from build123d import *

# Parameters (mm, degrees)
SKETCH2_W               = 76.2
SKETCH2_H               = 50.8
BOSS_EXTRUDE2_DEPTH     = 3.175
CUT_EXTRUDE1_DEPTH      = 63.861792847
CUT_EXTRUDE1_DEPTH_BACK = 63.861792847
CUT_EXTRUDE3_START      = -3.175
CUT_EXTRUDE3_DEPTH      = 3.175
CUT_EXTRUDE2_DEPTH      = 77.530014537
CUT_EXTRUDE2_DEPTH_BACK = 15.24
SKETCH4_R               = 1.27


with BuildPart() as part:
    # Sketch2 → Boss-Extrude2 (new, symmetric)
    with BuildSketch(Plane(origin=(0, 0, 0), x_dir=(0, 0, -1), z_dir=(1, 0, 0))):
        Polygon((-57.15, -6.35), (-57.15, -25.4), (-38.1, -25.4), (-38.1, 25.4), align=None)
        Rectangle(SKETCH2_W, SKETCH2_H)
    extrude(amount=BOSS_EXTRUDE2_DEPTH, both=True)

    # Sketch3 → Cut-Extrude1 (cut, two sides: drawn at the far end of the back side and taken through both)
    with BuildSketch(Plane(origin=(3.175, 0, 0), x_dir=(0, 0, -1), z_dir=(1, 0, 0)).offset(-CUT_EXTRUDE1_DEPTH_BACK)):
        with BuildLine():
            Line((-12.499999952, -9.525), (-12.499999952, 15.875))
            ThreePointArc((-12.499999952, 15.875), (-14, 17.375000048), (-15.500000048, 15.875))
            Line((-15.500000048, 15.875), (-15.500000048, -9.525))
            ThreePointArc((-15.500000048, -9.525), (-14, -11.025000048), (-12.499999952, -9.525))
        make_face()
        with BuildLine():
            Line((15.500000048, -9.525), (15.500000048, 15.875))
            ThreePointArc((15.500000048, 15.875), (14, 17.375000048), (12.499999952, 15.875))
            Line((12.499999952, 15.875), (12.499999952, -9.525))
            ThreePointArc((12.499999952, -9.525), (14, -11.025000048), (15.500000048, -9.525))
        make_face()
    extrude(amount=CUT_EXTRUDE1_DEPTH + CUT_EXTRUDE1_DEPTH_BACK, mode=Mode.SUBTRACT)

    # Sketch3_3 → Cut-Extrude3 (cut)
    # profile 1 of 2: a face of its own
    with BuildSketch(Plane(origin=(3.175, 0, 0), x_dir=(0, 0, -1), z_dir=(1, 0, 0)).offset(CUT_EXTRUDE3_START)):
        with BuildLine():
            Line((-18.250000009, -9.525), (-18.250000009, 15.875))
            ThreePointArc((-18.250000009, 15.875), (-14, 20.125000009), (-9.749999991, 15.875))
            Line((-9.749999991, 15.875), (-9.749999991, -9.525))
            ThreePointArc((-9.749999991, -9.525), (-14, -13.775000009), (-18.250000009, -9.525))
        make_face()
        with BuildLine():
            Line((-15.500000048, -9.525), (-15.500000048, 15.875))
            ThreePointArc((-15.500000048, 15.875), (-14, 17.375000048), (-12.499999952, 15.875))
            Line((-12.499999952, 15.875), (-12.499999952, -9.525))
            ThreePointArc((-12.499999952, -9.525), (-14, -11.025000048), (-15.500000048, -9.525))
        make_face(mode=Mode.SUBTRACT)
    # profile 2 of 2: a face of its own
    with BuildSketch(Plane(origin=(3.175, 0, 0), x_dir=(0, 0, -1), z_dir=(1, 0, 0)).offset(CUT_EXTRUDE3_START)):
        with BuildLine():
            Line((9.749999991, -9.525), (9.749999991, 15.875))
            ThreePointArc((9.749999991, 15.875), (14, 20.125000009), (18.250000009, 15.875))
            Line((18.250000009, 15.875), (18.250000009, -9.525))
            ThreePointArc((18.250000009, -9.525), (14, -13.775000009), (9.749999991, -9.525))
        make_face()
        with BuildLine():
            Line((12.499999952, -9.525), (12.499999952, 15.875))
            ThreePointArc((12.499999952, 15.875), (14, 17.375000048), (15.500000048, 15.875))
            Line((15.500000048, 15.875), (15.500000048, -9.525))
            ThreePointArc((15.500000048, -9.525), (14, -11.025000048), (12.499999952, -9.525))
        make_face(mode=Mode.SUBTRACT)
    extrude(amount=CUT_EXTRUDE3_DEPTH, mode=Mode.SUBTRACT)

    # Sketch4 → Cut-Extrude2 (cut, two sides: drawn at the far end of the back side and taken through both)
    with BuildSketch(Plane.XZ.offset(25.4).offset(-CUT_EXTRUDE2_DEPTH_BACK)):
        with Locations(Location((0, 25.4, 0), (0, 0, 90))):
            Circle(SKETCH4_R)
        with Locations(Location((0, 0, 0), (0, 0, 90))):
            Circle(SKETCH4_R)
        with Locations(Location((0, -25.4, 0), (0, 0, 90))):
            Circle(SKETCH4_R)
        with Locations(Location((0, 34.925, 0), (0, 0, 90))):
            Circle(SKETCH4_R)
        with Locations(Location((0, 44.45, 0), (0, 0, 90))):
            Circle(SKETCH4_R)
    extrude(amount=CUT_EXTRUDE2_DEPTH + CUT_EXTRUDE2_DEPTH_BACK, mode=Mode.SUBTRACT)


solid = part.part
The model under review builds one solid part; all positions refer to its coordinate system, in mm. A direction names the side the tool comes from. Round coordinates to 2 decimals unless told otherwise and drop trailing zeros. Loops run counter-clockwise (first coordinate to the right, second up) from the corner with the lowest first, then second, coordinate; pieces in that order, holes last. Notation, with made-up numbers: M 77,15.25 L 86,15.25 A23 cw 86,27.25 Z; hole C 55,20.25 d7. An arc over 180 degrees is marked long. Answer as a JSON object with one key per item and string values.
Item 1: For line 1 along Z through (x, y) = (1, 13.5); line 2 along X through (y, z) = (-21, 0) (3 decimals); line 3 along Z through (x, y) = (2.25, 10), list the stretches that pass through material, from the lowest coordinate up.
Check sheet entries:
{"line 1": "-38.1 to -18.25, -9.75 to 9.75, 18.25 to 45.24", "line 2": "-3.175 to -1.27, 1.27 to 3.175", "line 3": "-38.1 to -18.25, -9.75 to 9.75, 18.25 to 47.34"}
Item 2: We need section C-C, the plane y = -20. State the section outline as (x, z) points (3 decimals).
Check sheet entries:
{"outline": "M -3.175,-38.1 L 3.175,-38.1 L 3.175,57.15 L -3.175,57.15 Z; hole C 0,-25.4 d2.54; hole C 0,0 d2.54; hole C 0,25.4 d2.54; hole C 0,34.925 d2.54; hole C 0,44.45 d2.54"}
Item 3: We need section B-B, the plane z = 14. State the section outline as (x, y) points (3 decimals).
Check sheet entries:
{"outline": "M -3.175,-25.4 L 3.175,-25.4 L 3.175,-13.775 L 0,-13.775 L 0,-11.025 L -3.175,-11.025 Z; M -3.175,17.375 L 0,17.375 L 0,20.125 L 3.175,20.125 L 3.175,25.4 L -3.175,25.4 Z"}
Item 4: We need section D-D, the plane y = -4. State the section outline as (x, z) points (3 decimals), and give its area (3 significant figures).
Check sheet entries:
{"outline": "M -3.175,-38.1 L 3.175,-38.1 L 3.175,-18.25 L 0,-18.25 L 0,-15.5 L -3.175,-15.5 Z; M -3.175,-12.5 L 0,-12.5 L 0,-9.75 L 3.175,-9.75 L 3.175,9.75 L 0,9.75 L 0,12.5 L -3.175,12.5 Z; M -3.175,15.5 L 0,15.5 L 0,18.25 L 3.175,18.25 L 3.175,55.74 L -3.175,55.74 Z", "area": "523 mm2"}
Item 5: The part is to be moulded in two halves that separate along Y. For faces 5 (the face through (0, -10.16, 0)), 6 (the face through (-0.06, -17.67, 43.18)), 7 (the face through (2, 3, 9.75)), say which applies: +Y half, -Y half, draft (parallel to the pull), parting line (faces both ways), or undercut.
Check sheet entries:
{"face 5": "-Y half", "face 6": "draft", "face 7": "undercut"}
Item 6: Clearance check with flat-ended pins moving along their axes: P1, Ø1, axis at x = -1, y = -0.5, coming from the +Z side; P2, Ø3, axis at x = 1.5, z = 46, coming from the +Y side; P3, Ø0.8, axis at x = 0.5, z = 25.5, coming from the -Y side. State where each tip first meets the part, or that it passes through.
Check sheet entries:
{"P1": "z = 53.94", "P2": "y = 14.73", "P3": "y = -10.16"}
Item 7: Tool access review of faces 1 (the face through (0, 3, -12)), 2 (the face through (0, -16, 57.15)), 3 (the face through (0, -10.16, -25)), 4 (the face through (-1.61, 17.375, 13.967)): name each direction out of +Z, -Z, +X, -X, +Y, -Y from which nothing blocks a thin tool from reaching the whole face with its end or side.
Check sheet entries:
{"face 1": "+X", "face 2": "+Z, +X, -X, +Y, -Y", "face 3": "-Y", "face 4": "+X, -X"}
Item 8: We need section A-A, the plane y = 10. State the section outline as (x, z) points (3 decimals).
Check sheet entries:
{"outline": "M -3.175,-38.1 L 3.175,-38.1 L 3.175,-18.25 L 0,-18.25 L 0,-15.5 L -3.175,-15.5 Z; M -3.175,-12.5 L 0,-12.5 L 0,-9.75 L 3.175,-9.75 L 3.175,9.75 L 0,9.75 L 0,12.5 L -3.175,12.5 Z; M -3.175,15.5 L 0,15.5 L 0,18.25 L 3.175,18.25 L 3.175,47.34 L -3.175,47.34 Z"}
